Source: CAD feature listing. Evaluate the final solid. Frame: model axes, mm. A direction names the side the tool comes from. Coordinates: 2 decimals unless noted, no trailing zeros. Loops run counter-clockwise (first coordinate to the right, second up) from the corner with the lowest first, then second, coordinate; pieces in that order, holes last. Notation, with made-up numbers: M -26,30 L -15,30 A20 cw -15,50 Z; hole C 88.5,84.5 d5. An arc over 180 degrees is marked long. One line per question, with ' | ' between items. Start each with the question number.
1. Section query B-B, the plane z = 0. Output: boundary loops of the cut face in (x, y).
2. Pin query (flat end, axial travel): P1, Ø12, axis at x = -79.5, z = 14, coming from the +Y side; P2, Ø6, axis at x = -25.5, y = -18.5, coming from the -Z side; P3, Ø6, axis at x = 4.5, y = 14.5, coming from the +Z side. Return the tip coordinate at first contact, or that it passes through.
3. Section query A-A, the plane x = 0. Output: boundary loops of the cut face in (y, z).
4. Section query C-C, the plane x = -49. Output: boundary loops of the cut face in (y, z).
5. Mould query, pull axis X, two halves, no side actions, for faces 1 (the flat face through (-71.754, 0.455, 60.841)), 2 (the cylindrical face through (-70.623, 0.455, 47.301)), 3 (the cylindrical face through (39.344, 0.455, 95.185)), 4 (the cylindrical face through (-70.727, 0.455, -47.146)). Classes: pulls with the +X half, pulls with the -X half, needs draft (parallel to the pull), parting line crosses it, or undercut.
6. Ray query, probe 1 along X at (y, z) = (-7.5, 0); probe 2 along X at (y, z) = (-21, -92.5); probe 3 along Z at (x, y) = (-90, -12). Return the intervals inside material, ascending.
7. Access query for faces 5 (the flat face through (60.841, 0.455, 71.754)), 6 (the flat face through (47, 32.5, -47)), 7 (the cylindrical face through (-47.301, 0.455, -70.623)), 8 (the flat face through (7.717, 0.455, -93.758)), 9 (the cylindrical face through (-83.385, 0.455, -16.491)). Directions: +Z, -Z, +X, -X, +Y, -Y. A direction counts if a zero-diameter tool reaches every point of the face in a straight line with its end or side. Return the directions, or none.
```python
from build123d import *

# Parameters (mm, degrees)
SKETCH1_R           = 105
BOSS_EXTRUDE1_DEPTH = 32.5
SKETCH2_R           = 62.5
BOSS_EXTRUDE2_DEPTH = 38.75
CUT_EXTRUDE1_DEPTH  = 168.5
CUT_EXTRUDE2_DEPTH  = 165.70143442
SKETCH5_R           = 105
SKETCH5_R_2         = 102.995839741
CUT_EXTRUDE3_DEPTH  = 165.70143442


with BuildPart() as part:
    # Sketch1 → Boss-Extrude1 (new, symmetric)
    with BuildSketch(Plane(origin=(0, 0, 0), x_dir=(1, 0, 0), z_dir=(0, 1, 0))):
        with Locations(Location((0, 0, 0), (0, 0, 270))):
            Circle(SKETCH1_R)
    extrude(amount=BOSS_EXTRUDE1_DEPTH, both=True)

    # Sketch2 → Boss-Extrude2 (add, symmetric)
    with BuildSketch(Plane(origin=(0, 0, 0), x_dir=(1, 0, 0), z_dir=(0, 1, 0))):
        with Locations(Location((0, 0, 0), (0, 0, 270))):
            Circle(SKETCH2_R)
    extrude(amount=BOSS_EXTRUDE2_DEPTH, both=True)

    # Sketch3 → Cut-Extrude1 (cut, through all)
    with BuildSketch(Plane(origin=(0, 38.75, 0), x_dir=(1, 0, 0), z_dir=(0, 1, 0))):
        with BuildLine():
            Line((-10, 43.874821937), (-10, 51.374821937))
            Line((-10, 51.374821937), (10, 51.374821937))
            Line((10, 51.374821937), (10, 43.874821937))
            ThreePointArc((10, 43.874821937), (0, -45), (-10, 43.874821937))
        make_face()
    extrude(amount=-CUT_EXTRUDE1_DEPTH, mode=Mode.SUBTRACT)

    # Sketch4 → Cut-Extrude2 (cut, through all)
    with BuildSketch(Plane(origin=(0, 32.5, 0), x_dir=(1, 0, 0), z_dir=(0, 1, 0))):
        with BuildLine():
            Line((-5, 104.880884817), (-10, 84.409715081))
            ThreePointArc((-10, 84.409715081), (-16.582677371, 83.366748834), (-23.063404167, 81.811242432))
            Line((-23.063404167, 81.811242432), (-35.516779329, 98.810719996))
            ThreePointArc((-35.516779329, 98.810719996), (-20.484483812, 102.982454442), (-5, 104.880884817))
        make_face()
        with BuildLine():
            Line((5, 104.880884817), (10, 84.409715081))
            ThreePointArc((10, 84.409715081), (16.582677371, 83.366748834), (23.063404167, 81.811242432))
            Line((23.063404167, 81.811242432), (35.516779329, 98.810719996))
            ThreePointArc((35.516779329, 98.810719996), (20.484483812, 102.982454442), (5, 104.880884817))
        make_face()
        with BuildLine():
            Line((44.755574654, 94.983885672), (41.540994817, 74.157573784))
            ThreePointArc((41.540994817, 74.157573784), (47.223469807, 70.674917046), (52.61561412, 66.757749743))
            Line((52.61561412, 66.757749743), (70.626450965, 77.697518777))
            ThreePointArc((70.626450965, 77.697518777), (58.334874467, 87.304309292), (44.755574654, 94.983885672))
        make_face()
        with BuildLine():
            Line((77.697518777, 70.626450965), (66.757749743, 52.61561412))
            ThreePointArc((66.757749743, 52.61561412), (70.674917046, 47.223469807), (74.157573784, 41.540994817))
            Line((74.157573784, 41.540994817), (94.983885672, 44.755574654))
            ThreePointArc((94.983885672, 44.755574654), (87.304309292, 58.334874467), (77.697518777, 70.626450965))
        make_face()
        with BuildLine():
            Line((98.810719996, 35.516779329), (81.811242432, 23.063404167))
            ThreePointArc((81.811242432, 23.063404167), (83.366748834, 16.582677371), (84.409715081, 10))
            Line((84.409715081, 10), (104.880884817, 5))
            ThreePointArc((104.880884817, 5), (102.982454442, 20.484483812), (98.810719996, 35.516779329))
        make_face()
        with BuildLine():
            Line((104.880884817, -5), (84.409715081, -10))
            ThreePointArc((84.409715081, -10), (83.366748834, -16.582677371), (81.811242432, -23.063404167))
            Line((81.811242432, -23.063404167), (98.810719996, -35.516779329))
            ThreePointArc((98.810719996, -35.516779329), (102.982454442, -20.484483812), (104.880884817, -5))
        make_face()
        with BuildLine():
            Line((94.983885672, -44.755574654), (74.157573784, -41.540994817))
            ThreePointArc((74.157573784, -41.540994817), (70.674917046, -47.223469807), (66.757749743, -52.61561412))
            Line((66.757749743, -52.61561412), (77.697518777, -70.626450965))
            ThreePointArc((77.697518777, -70.626450965), (87.304309292, -58.334874467), (94.983885672, -44.755574654))
        make_face()
        with BuildLine():
            Line((70.626450965, -77.697518777), (52.61561412, -66.757749743))
            ThreePointArc((52.61561412, -66.757749743), (47.223469807, -70.674917046), (41.540994817, -74.157573784))
            Line((41.540994817, -74.157573784), (44.755574654, -94.983885672))
            ThreePointArc((44.755574654, -94.983885672), (58.334874467, -87.304309292), (70.626450965, -77.697518777))
        make_face()
        with BuildLine():
            Line((35.516779329, -98.810719996), (23.063404167, -81.811242432))
            ThreePointArc((23.063404167, -81.811242432), (16.582677371, -83.366748834), (10, -84.409715081))
            Line((10, -84.409715081), (5, -104.880884817))
            ThreePointArc((5, -104.880884817), (20.484483812, -102.982454442), (35.516779329, -98.810719996))
        make_face()
        with BuildLine():
            Line((-5, -104.880884817), (-10, -84.409715081))
            ThreePointArc((-10, -84.409715081), (-16.582677371, -83.366748834), (-23.063404167, -81.811242432))
            Line((-23.063404167, -81.811242432), (-35.516779329, -98.810719996))
            ThreePointArc((-35.516779329, -98.810719996), (-20.484483812, -102.982454442), (-5, -104.880884817))
        make_face()
        with BuildLine():
            Line((-44.755574654, -94.983885672), (-41.540994817, -74.157573784))
            ThreePointArc((-41.540994817, -74.157573784), (-47.223469807, -70.674917046), (-52.61561412, -66.757749743))
            Line((-52.61561412, -66.757749743), (-70.626450965, -77.697518777))
            ThreePointArc((-70.626450965, -77.697518777), (-58.334874467, -87.304309292), (-44.755574654, -94.983885672))
        make_face()
        with BuildLine():
            Line((-77.697518777, -70.626450965), (-66.757749743, -52.61561412))
            ThreePointArc((-66.757749743, -52.61561412), (-70.674917046, -47.223469807), (-74.157573784, -41.540994817))
            Line((-74.157573784, -41.540994817), (-94.983885672, -44.755574654))
            ThreePointArc((-94.983885672, -44.755574654), (-87.304309292, -58.334874467), (-77.697518777, -70.626450965))
        make_face()
        with BuildLine():
            Line((-98.810719996, -35.516779329), (-81.811242432, -23.063404167))
            ThreePointArc((-81.811242432, -23.063404167), (-83.366748834, -16.582677371), (-84.409715081, -10))
            Line((-84.409715081, -10), (-104.880884817, -5))
            ThreePointArc((-104.880884817, -5), (-102.982454442, -20.484483812), (-98.810719996, -35.516779329))
        make_face()
        with BuildLine():
            Line((-104.880884817, 5), (-84.409715081, 10))
            ThreePointArc((-84.409715081, 10), (-83.366748834, 16.582677371), (-81.811242432, 23.063404167))
            Line((-81.811242432, 23.063404167), (-98.810719996, 35.516779329))
            ThreePointArc((-98.810719996, 35.516779329), (-102.982454442, 20.484483812), (-104.880884817, 5))
        make_face()
        with BuildLine():
            Line((-94.983885672, 44.755574654), (-74.157573784, 41.540994817))
            ThreePointArc((-74.157573784, 41.540994817), (-70.674917046, 47.223469807), (-66.757749743, 52.61561412))
            Line((-66.757749743, 52.61561412), (-77.697518777, 70.626450965))
            ThreePointArc((-77.697518777, 70.626450965), (-87.304309292, 58.334874467), (-94.983885672, 44.755574654))
        make_face()
        with BuildLine():
            Line((-70.626450965, 77.697518777), (-52.61561412, 66.757749743))
            ThreePointArc((-52.61561412, 66.757749743), (-47.223469807, 70.674917046), (-41.540994817, 74.157573784))
            Line((-41.540994817, 74.157573784), (-44.755574654, 94.983885672))
            ThreePointArc((-44.755574654, 94.983885672), (-58.334874467, 87.304309292), (-70.626450965, 77.697518777))
        make_face()
    extrude(amount=-CUT_EXTRUDE2_DEPTH, mode=Mode.SUBTRACT)

    # Sketch5 → Cut-Extrude3 (cut, through all)
    with BuildSketch(Plane(origin=(0, 32.5, 0), x_dir=(1, 0, 0), z_dir=(0, 1, 0))):
        Circle(SKETCH5_R)
        Circle(SKETCH5_R_2, mode=Mode.SUBTRACT)
    extrude(amount=-CUT_EXTRUDE3_DEPTH, mode=Mode.SUBTRACT)


solid = part.part
```
Taken from the geometry:
1) outline: M -103,-32.5 L -62.5,-32.5 L -62.5,-38.75 L -45,-38.75 L -45,38.75 L -62.5,38.75 L -62.5,32.5 L -103,32.5 Z; M 45,-38.75 L 62.5,-38.75 L 62.5,-32.5 L 103,-32.5 L 103,32.5 L 62.5,32.5 L 62.5,38.75 L 45,38.75 Z
2) P1: y = 32.5 | P2: z = -89.23 | P3: z = 102.98
3) outline: M -38.75,-62.5 L -32.5,-62.5 L -32.5,-103 L 32.5,-103 L 32.5,-62.5 L 38.75,-62.5 L 38.75,-51.37 L -38.75,-51.37 Z; M -38.75,45 L 38.75,45 L 38.75,62.5 L 32.5,62.5 L 32.5,103 L -32.5,103 L -32.5,62.5 L -38.75,62.5 Z
4) outline: M -38.75,-38.8 L -32.5,-38.8 L -32.5,-69.46 L 32.5,-69.46 L 32.5,-38.8 L 38.75,-38.8 L 38.75,38.8 L 32.5,38.8 L 32.5,69.46 L -32.5,69.46 L -32.5,38.8 L -38.75,38.8 Z
5) face 1: pulls with the -X half | face 2: undercut | face 3: pulls with the +X half | face 4: undercut
6) probe 1: -103 to -45, 45 to 103 | probe 2: -44.37 to -30.89, -8.02 to 8.02, 30.89 to 44.37 | probe 3: -43.99 to -29.06, -8.63 to 8.63, 29.06 to 43.99
7) face 5: +Z, +Y, -Y | face 6: +Y | face 7: +Y, -Y | face 8: -Z, +Y, -Y | face 9: -X, +Y, -Y
